Work out the finished part from the listing and answer in its coordinate system (mm). A direction names the side the tool comes from. Round coordinates to 2 decimals unless told otherwise and drop trailing zeros. Write each loop counter-clockwise with the first axis right and the second up, starting at its lowest first coordinate (ties: lowest second). Pieces come first, ordered by that corner, then holes. Notation, with made-up numbers: (27.5, 4) - (65.5, 4) arc R19 ccw to (65.5, 13) - close; hole circle Ø1 at (11, -38.75). An arc over 180 degrees is marked (long way). Answer as a JSON object with one key per item and string values.
```python
from build123d import *

# Parameters (mm, degrees)
SKETCH1_R           = 116
BOSS_EXTRUDE1_DEPTH = 20
SKETCH2_R           = 10
BOSS_EXTRUDE2_DEPTH = 100
SKETCH3_OUTSIDE_W   = 303.87
SKETCH3_OUTSIDE_H   = 303.87
SKETCH3_OUTSIDE_R   = 7.5
CUT_EXTRUDE1_DEPTH  = 20


with BuildPart() as part:
    # Sketch1 → Boss-Extrude1 (new body)
    with BuildSketch(Plane(origin=(0, 0, 0), x_dir=(1, 0, 0), z_dir=(0, 1, 0))):
        with Locations(Location((0, 0, 0), (0, 0, 270))):
            Circle(SKETCH1_R)
    extrude(amount=BOSS_EXTRUDE1_DEPTH)

    # Sketch2 → Boss-Extrude2 (add)
    with BuildSketch(Plane(origin=(0, 20, 0), x_dir=(1, 0, 0), z_dir=(0, 1, 0))):
        with Locations(Location((0, 0, 0), (0, 0, 270))):
            Circle(SKETCH2_R)
    extrude(amount=BOSS_EXTRUDE2_DEPTH)

    # Sketch3 outside → Cut-Extrude1 (cut)
    with BuildSketch(Plane(origin=(0, 120, 0), x_dir=(1, 0, 0), z_dir=(0, 1, 0))):
        Rectangle(SKETCH3_OUTSIDE_W, SKETCH3_OUTSIDE_H)
        with Locations(Location((0, 0, 0), (0, 0, 270))):
            Circle(SKETCH3_OUTSIDE_R, mode=Mode.SUBTRACT)
    extrude(amount=-CUT_EXTRUDE1_DEPTH, mode=Mode.SUBTRACT)


solid = part.part
```
Item 1: A cutting plane is placed at B-B (z = 0). Write down the section's boundary in (x, y), and give its area (3 significant figures).
Results found:
{"outline": "(-116, 0) - (116, 0) - (116, 20) - (10, 20) - (10, 100) - (7.5, 100) - (7.5, 120) - (-7.5, 120) - (-7.5, 100) - (-10, 100) - (-10, 20) - (-116, 20) - close", "area": "6,540 mm²"}
Item 2: For faces 1 (the flat face through (4, 100, -7)), 2 (the flat face through (0, 120, 0)), determine the directions among +Z, -Z, +X, -X, +Y, -Y from which every point of the face is accessible in a straight line to the end or side of a thin tool.
Results found:
{"face 1": "+Y", "face 2": "+Z, -Z, +X, -X, +Y"}
Item 3: This flat-tipped pin is pushed along its axis until it touches: P1, Ø10, axis at x = 35.5, z = 22, coming from the +Y side. Where does it stop, or does it pass through?
Results found:
{"P1": "y = 20"}
Item 4: A cutting plane is placed at C-C (y = 112). Write down the section's boundary in (x, z).
Results found:
{"outline": "circle Ø15 at (0, 0)"}
Item 5: Consider line 1 along Y through (x, z) = (14, -101); line 2 along Z through (x, y) = (-30.5, 6.5); line 3 along X through (y, z) = (91, -3). Determine where each line is inside the solid, lowest interval first.
Results found:
{"line 1": "0 to 20", "line 2": "-111.92 to 111.92", "line 3": "-9.54 to 9.54"}
Item 6: A cutting plane is placed at D-D (y = 15.5). Write down the section's boundary in (x, z).
Results found:
{"outline": "circle Ø232 at (0, 0)"}
Item 7: A cutting plane is placed at A-A (x = 0). Write down the section's boundary in (y, z).
Results found:
{"outline": "(0, -116) - (20, -116) - (20, -10) - (100, -10) - (100, -7.5) - (120, -7.5) - (120, 7.5) - (100, 7.5) - (100, 10) - (20, 10) - (20, 116) - (0, 116) - close"}
